from build123d import *

# Parameters (mm, degrees)
SKETCH1_R           = 2.5
BOSS_EXTRUDE1_DEPTH = 27.5
BOSS_EXTRUDE2_START = -2
SKETCH2_R           = 4.25
SKETCH2_R_2         = 2.5
BOSS_EXTRUDE2_DEPTH = 2
SCALE1_SCALE        = 1.5


with BuildPart() as part:
    # Sketch1 → Boss-Extrude1 (new body)
    with BuildSketch(Plane(origin=(0, 0, 0), x_dir=(0, 0, -1), z_dir=(1, 0, 0))):
        Circle(SKETCH1_R)
    extrude(amount=BOSS_EXTRUDE1_DEPTH)

    # Sketch2 → Boss-Extrude2 (add)
    with BuildSketch(Plane(origin=(27.5, 0, 0), x_dir=(0, 0, -1), z_dir=(1, 0, 0)).offset(BOSS_EXTRUDE2_START)):
        Circle(SKETCH2_R)
        Circle(SKETCH2_R_2, mode=Mode.SUBTRACT)
    extrude(amount=BOSS_EXTRUDE2_DEPTH)


with BuildPart() as part_1:
    # Scale1: scaled about (15.29076087, 0, 0)
    add(part.part.scale(SCALE1_SCALE).moved(Location((-7.645380435, 0, 0))))


solid = part_1.part
Source: CAD feature listing. Evaluate the final solid. Frame: model axes, mm. A direction names the side the tool comes from. Round coordinates to 2 decimals unless told otherwise and drop trailing zeros. Loops run counter-clockwise (first coordinate to the right, second up) from the corner with the lowest first, then second, coordinate; pieces in that order, holes last. Notation, with made-up numbers: (27, 32.5) - (33, 32.5) arc R22 cw to (33, 65.5) - close; hole circle Ø5 at (-2.75, 57). An arc over 180 degrees is marked (long way). Write item = value, one per line. Start each with the question number.
(1) Ray query, line 1 along X through (y, z) = (-2.25, -4.75); line 2 along Y through (x, z) = (18, 0); line 3 along Y through (x, z) = (13.5, -3). Return the intervals inside material, ascending. Write a range as from..to.
(2) Pin query (flat end, axial travel): pin 1 (1 mm diameter, centred on x = 18.5, y = -3.5, fed in from +Z); pin 2 (4 mm diameter, centred on x = 23.5, z = -4.5, fed in from +Y); pin 3 (3 mm diameter, centred on x = -1, z = -2.5, fed in from -Y). Return the tip coordinate at first contact, or that it passes through.
(3) Set-up query: faces 1 (the face through (33.605, 0, 0)), 2 (the face through (11.212, 0.165, 3.746)). Return all of +Z, -Z, +X, -X, +Y, -Y with unobstructed straight access to the full face (end or side cutting, diameter ignored); none if empty.
(4) Section query C-C, the plane x = 9. Output: boundary loops of the cut face in (y, z), plus the area to 3 significant figures.
(5) Section query A-A, the plane y = 0. Output: boundary loops of the cut face in (x, z) (3 decimals).
(6) Section query D-D, the plane x = 31. Output: boundary loops of the cut face in (y, z) (3 decimals), plus the area to 3 significant figures.
Conclusion:
q1.line_1 = 30.6..33.6
q1.line_2 = -3.75..3.75
q1.line_3 = -2.25..2.25
q2.pin_1 = 2.25
q2.pin_2 = 2.8
q2.pin_3 = -3.61
q3.face_1 = +Z, -Z, +X, +Y, -Y
q3.face_2 = -X
q4.outline = circle Ø7.5 at (0, 0)
q4.area = 44.2 mm2
q5.outline = (-7.645, -3.75) - (30.605, -3.75) - (30.605, -6.375) - (33.605, -6.375) - (33.605, 6.375) - (30.605, 6.375) - (30.605, 3.75) - (-7.645, 3.75) - close
q6.outline = circle Ø12.75 at (0, 0)
q6.area = 128 mm2
